```python
from build123d import *

# Parameters (mm, degrees)
F1_DEPTH      = 120
F1_DEPTH_BACK = 120
F2_R          = 3
F4_DEPTH      = 30.001
F6_D          = 4.2


with BuildPart() as f1:
    # F0 (on Right) → F1 (new body, two sides)
    with BuildSketch(Plane.YZ) as f1_sk:
        Polygon((0, 0), (0, -30), (3, -30), (3, -3), (30, -3), (30, 0), align=None)
    extrude(amount=F1_DEPTH)
    extrude(f1_sk.sketch, amount=-F1_DEPTH_BACK)

    # F2
    f2_edges = [f1.edges().sort_by_distance(p)[0] for p in [
        (0, 3, -3),
    ]]
    fillet(f2_edges, radius=F2_R)

    # F3 (on face) → F4 (cut, through all)
    with BuildSketch(Plane.XZ):
        Polygon((-80, -40), (-130, 10), (-130, -40), align=None)
        Polygon((130, -40), (130, 10), (80, -40), align=None)
    extrude(amount=-F4_DEPTH, mode=Mode.SUBTRACT)

    # F6 (through all)
    with Locations(Plane.XY):
        with Locations((-87, 21), (-65, 21)):
            Hole(F6_D / 2)


solid = f1.part
```
The listing builds one solid part. Answer for the finished solid, in the listing's coordinates (mm). A direction names the side the tool comes from. Round coordinates to 2 decimals unless told otherwise and drop trailing zeros. Order: outer loops, then holes, each group sorted by start corner. A loop starts at its lowest first (then second) coordinate and runs counter-clockwise, first axis right, second up. Notation, with made-up numbers: (-34.5, -19.5) - (-11.5, -19.5) arc R13 cw to (-11.5, -11.5) - close; hole circle Ø10 at (-19, -12.5). An arc over 180 degrees is marked (long way). Put each result on its own line as item: value. Start each with the question number.
(1) Straight lines are drawn through the part: probe 1 along Y at (x, z) = (-87, -1.25); probe 2 along Z at (x, y) = (93, 26.5); probe 3 along Y at (x, z) = (38, -27.5). For each, find the intervals that lie inside material, in ascending order. Write a range as from..to.
(2) Given P1, Ø6, axis at x = 11.5, y = 17, coming from the -Z side; P2, Ø12, axis at x = -43.5, z = -9.5, coming from the +Y side; P3, Ø4, axis at y = 3.5, z = -12, coming from the -X side, each flat-ended and moving along its own axis, determine where each tip first touches the part or whether it passes through.
(3) Find section C-C (z = -21). Give the vertices of the cut face in (x, y).
(4) Find section A-A (x = -65). Give the vertices of the cut face in (y, z), plus the area to 3 significant figures.
(5) Find section B-B (y = 21). Give the vertices of the cut face in (x, z), plus the area to 3 significant figures.
(6) For faces 4 (the flat face through (2, 3, -18)), 5 (the cylindrical face through (-67.003, 21.631, -1.521)), determine the directions among +Z, -Z, +X, -X, +Y, -Y from which every point of the face is accessible in a straight line to the end or side of a thin tool.
(7) Determine the mould class of faces 1 (the cylindrical face through (-84.9, 21.09, -1.52)), 2 (the flat face through (-110.5, 2.7, -9.5)), 3 (the flat face through (2, 15, 0)) for opening direction X: released by +X, released by -X, zero draft, split by the parting line, or undercut.
Reply:
1. probe 1: 0..18.9, 23.1..30
1. probe 2: -3..0
1. probe 3: 0..3
2. P1: z = -3
2. P2: y = 4.34
2. P3: x = -109.94
3. outline: (-99, 0) - (99, 0) - (99, 3) - (-99, 3) - close
4. outline: (0, -30) - (3, -30) - (3, -6) arc R3 cw to (6, -3) - (18.9, -3) - (18.9, 0) - (0, 0) - close; (23.1, -3) - (30, -3) - (30, 0) - (23.1, 0) - close
4. area: 160 mm^2
5. outline: (-120, 0) - (-117, -3) - (-89.1, -3) - (-89.1, 0) - close; (-84.9, -3) - (-67.1, -3) - (-67.1, 0) - (-84.9, 0) - close; (-62.9, -3) - (117, -3) - (120, 0) - (-62.9, 0) - close
5. area: 686 mm^2
6. face 4: -Z, +X, -X, +Y
6. face 5: +Z, -Z
7. face 1: undercut
7. face 2: released by -X
7. face 3: zero draft
